Model file for the job. Use its own axes, mm. A direction names the side the tool comes from. Round coordinates to 2 decimals unless told otherwise and drop trailing zeros. Order: outer loops, then holes, each group sorted by start corner. A loop starts at its lowest first (then second) coordinate and runs counter-clockwise, first axis right, second up. Notation, with made-up numbers: (41, 76.5) -> (45, 76.5) arc R7 cw to (45, 86.5) -> close; hole circle Ø11 at (57.5, 77.25). An arc over 180 degrees is marked (long way). Use CSV: the item, a comma, the result in double quotes.
```python
from build123d import *

# Parameters (mm, degrees)
F0_R     = 41.275
F0_R_2   = 3.175
F1_DEPTH = 38.1
F2_R     = 3.175
F3_DEPTH = 38.101
F4_R     = 9.525
F4_R_2   = 3.175
F5_DEPTH = 6.35
F6_R     = 9.525
F7_DEPTH = 6.35


with BuildPart() as f1:
    # F0 (on Front) → F1 (new body)
    with BuildSketch(Plane.XZ):
        Circle(F0_R)
        Circle(F0_R_2, mode=Mode.SUBTRACT)
    extrude(amount=F1_DEPTH)

    # F2 (on face) → F3 (cut, through all)
    with BuildSketch(Plane.XZ.offset(38.1)):
        with Locations((0, 31.75)):
            Circle(F2_R)
    extrude(amount=-F3_DEPTH, mode=Mode.SUBTRACT)

    # F4 (on face) → F5 (cut)
    with BuildSketch(Plane(origin=(0, 0, 0), x_dir=(-1, 0, 0), z_dir=(0, 1, 0))):
        Circle(F4_R)
        Circle(F4_R_2, mode=Mode.SUBTRACT)
    extrude(amount=-F5_DEPTH, mode=Mode.SUBTRACT)

    # F6 (on face) → F7 (cut)
    with BuildSketch(Plane.XZ.offset(38.1)):
        Circle(F6_R)
    extrude(amount=-F7_DEPTH, mode=Mode.SUBTRACT)


solid = f1.part
```
Q1. Mould opens along Z. For faces 4 (the cylindrical face through (-8.948, -18.783, -40.293)), 5 (the flat face through (-1, -38.1, 10)), 6 (the cylindrical face through (-0.69, -18.87, -3.1)) say: +Z half, -Z half, draft (parallel to the pull), parting line (faces both ways), or undercut.
From the geometry:
face 4,"parting line"
face 5,"draft"
face 6,"undercut"
Q2. Cut at B-B (z = 0). Give the cut face in (x, y) (3 decimals), plus the area to 3 significant figures.
From the geometry:
outline,"(-41.275, -38.1) -> (-9.525, -38.1) -> (-9.525, -31.75) -> (-3.175, -31.75) -> (-3.175, -6.35) -> (-9.525, -6.35) -> (-9.525, 0) -> (-41.275, 0) -> close; (3.175, -31.75) -> (9.525, -31.75) -> (9.525, -38.1) -> (41.275, -38.1) -> (41.275, 0) -> (9.525, 0) -> (9.525, -6.35) -> (3.175, -6.35) -> close"
area,"2,740 mm²"
Q3. Cut at D-D (z = 31.75). Give the cut face in (x, y) (3 decimals).
From the geometry:
outline,"(-26.374, -38.1) -> (-3.175, -38.1) -> (-3.175, 0) -> (-26.374, 0) -> close; (3.175, -38.1) -> (26.374, -38.1) -> (26.374, 0) -> (3.175, 0) -> close"
Q4. Probe line 1 along Z through (x, y) = (0, -17.25) (3 decimals); line 2 along Z through (x, y) = (0, -4) (3 decimals); line 3 along Z through (x, y) = (-4.5, -34). List the from-to ranges inside material, lowest first.
From the geometry:
line 1,"z = -41.275 to -3.175, 3.175 to 28.575, 34.925 to 41.275"
line 2,"z = -41.275 to -9.525, 9.525 to 28.575, 34.925 to 41.275"
line 3,"z = -41.03 to -8.39, 8.39 to 41.03"
Q5. Cut at A-A (x = 0). Give the cut face in (y, z) (3 decimals), plus the area to 3 significant figures.
From the geometry:
outline,"(-38.1, -41.275) -> (0, -41.275) -> (0, -9.525) -> (-6.35, -9.525) -> (-6.35, -3.175) -> (-31.75, -3.175) -> (-31.75, -9.525) -> (-38.1, -9.525) -> close; (-38.1, 9.525) -> (-31.75, 9.525) -> (-31.75, 3.175) -> (-6.35, 3.175) -> (-6.35, 9.525) -> (0, 9.525) -> (0, 28.575) -> (-38.1, 28.575) -> close; (-38.1, 34.925) -> (0, 34.925) -> (0, 41.275) -> (-38.1, 41.275) -> close"
area,"2,500 mm²"
Q6. Pin check, flat tips, straight feed: pin 1 (1 mm diameter, centred on y = -21.5, z = -12.5, fed in from +X); pin 2 (17 mm diameter, centred on x = 0, z = 0, fed in from +Y); pin 3 (1 mm diameter, centred on x = 12.5, y = -10, fed in from +Z); pin 4 (5 mm diameter, centred on x = -7, z = 2.5, fed in from +Y). Stop position of each tip, or through.
From the geometry:
pin 1,"stops at x = 39.49"
pin 2,"stops at y = -6.35"
pin 3,"stops at z = 39.49"
pin 4,"stops at y = 0"
Q7. Which spindle directions (+Z, -Z, +X, -X, +Y, -Y) get a long thin tool onto all of the face, cutting with end or side? Do faces 1 (the cylindrical face through (-7.559, -34.969, -5.796)), 2 (the cylindrical face through (-0.69, -19.32, 28.65)), 3 (the flat face through (-4, -6.35, 0)). Say none if no direction does.
From the geometry:
face 1,"-Y"
face 2,"+Y, -Y"
face 3,"+Y"
Q8. Cut at C-C (y = -13). Give the cut face in (x, z) (3 decimals), plus the area to 3 significant figures.
From the geometry:
outline,"circle Ø82.55 at (0, 0); hole circle Ø6.35 at (0, 0); hole circle Ø6.35 at (0, 31.75)"
area,"5,290 mm²"
